Part print with two shaded views. Sizes in mm from the minimum x, y, z corner. Give positions to 0.01 mm unless a question says otherwise; leave off trailing zeros. Order: outer loops, then holes, each group sorted by start corner. A loop starts at its lowest first (then second) coordinate and runs counter-clockwise, first axis right, second up. Notation, with made-up numbers: M 8,29.5 L 17,29.5 A7 ccw 17,41.5 Z; hole C 10,25.5 d3. An arc over 180 degrees is marked long. Return JSON: item names as keys, results as strings. Group by question number.
1. Slice it at C-C on x = 211. List the corners of the cut face in (y, z).
2. Slice it at A-A on z = 15. List the corners of the cut face in (x, y), then the cut area to 3 significant figures.
3. Wall check: probe 1 along X at (y, z) = (23, 10.5); probe 2 along Z at (x, y) = (160.5, 15.5); probe 3 along Y at (x, z) = (308, 10.5). Give the ranges that are in metal, low to high. Write a range as [from, to].
4. Pin check, flat tips, straight feed: pin 1 (4 mm diameter, centred on x = 350.5, z = 20.5, fed in from -Y); pin 2 (5 mm diameter, centred on x = 240, z = 5, fed in from +Y); pin 3 (1.5 mm diameter, centred on x = 205, z = 10.5, fed in from -Y). Stop position of each tip, or through.
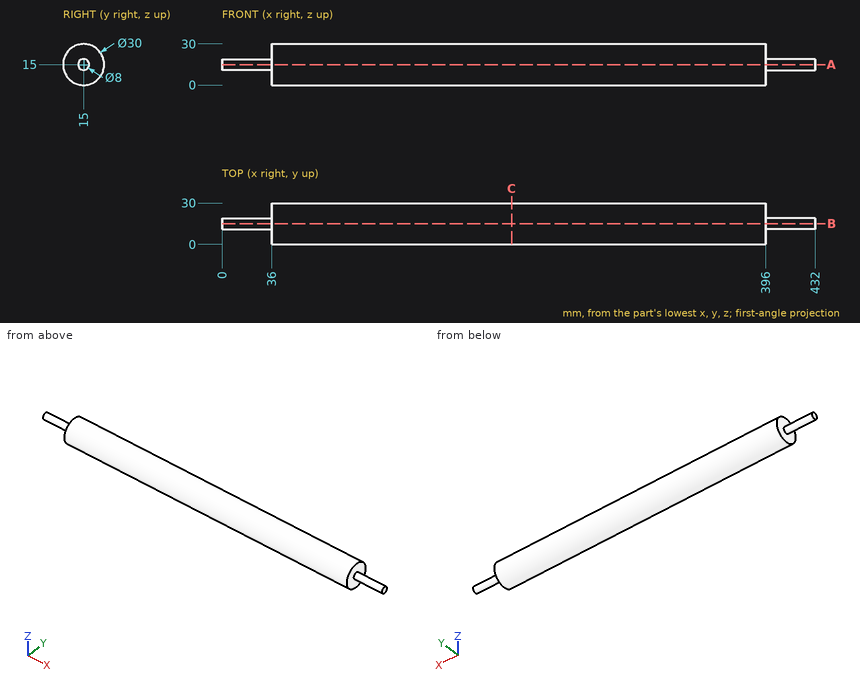
Result:
{
 "1": {"outline": "C 15,15 d30"},
 "2": {"outline": "M 0,11 L 36,11 L 36,0 L 396,0 L 396,11 L 432,11 L 432,19 L 396,19 L 396,30 L 36,30 L 36,19 L 0,19 Z", "area": "11,400 mm2"},
 "3": {"probe 1": "x = [36, 396]", "probe 2": "z = [0.01, 29.99]", "probe 3": "y = [0.69, 29.31]"},
 "4": {"pin 1": "stops at y = 0.41", "pin 2": "stops at y = 27.99", "pin 3": "stops at y = 0.48"}
}
